Verification items for this drawing (mm, ordinates from the low corner). A direction names the side the tool comes from. Round coordinates to 2 decimals unless told otherwise and drop trailing zeros. Write each loop counter-clockwise with the first axis right and the second up, starting at its lowest first coordinate (ties: lowest second). Pieces come first, ordered by that corner, then holes.
Item 1: Scan lines: probe 1 along X at (y, z) = (4.5, 21); probe 2 along Y at (x, z) = (37.5, 40); probe 3 along X at (y, z) = (9, 9) (1 decimal). Record each from-to range of solid material in increasing order.
Item 2: Cross-section at D-D (x = 5). Enter the section's corners in (y, z), then the cut area to 3 significant figures.
Item 3: Cross-section at A-A (y = 5.5). Enter the section's corners in (x, z), then the cut area to 3 significant figures.
Item 4: Access from +Z, -Z, +X, -X, +Y, -Y to the whole of each face (thin tool, end or side, straight path). Record for the marked faces 1, 2 and 3.
Item 5: Draft check along X on the marked faces 4, 5 and 6. Enter one of: pulls with the +X half, pulls with the -X half, needs draft (parallel to the pull), parting line crosses it, or undercut.
Item 6: Cross-section at B-B (x = 26.25). Enter the section's corners in (y, z).
Item 7: Cross-section at C-C (z = 14). Enter the section's corners in (x, y) (1 decimal).
Item 8: Depth check by flat-ended pin: P1, Ø2.5, axis at x = 47, y = 14, coming from the -Z side; P2, Ø1, axis at x = 5, y = 14, coming from the +Z side; P3, Ø3.5, axis at y = 4.5, z = 6.5, coming from the -X side. Enter the tip coordinate at first touch or a pass-through.
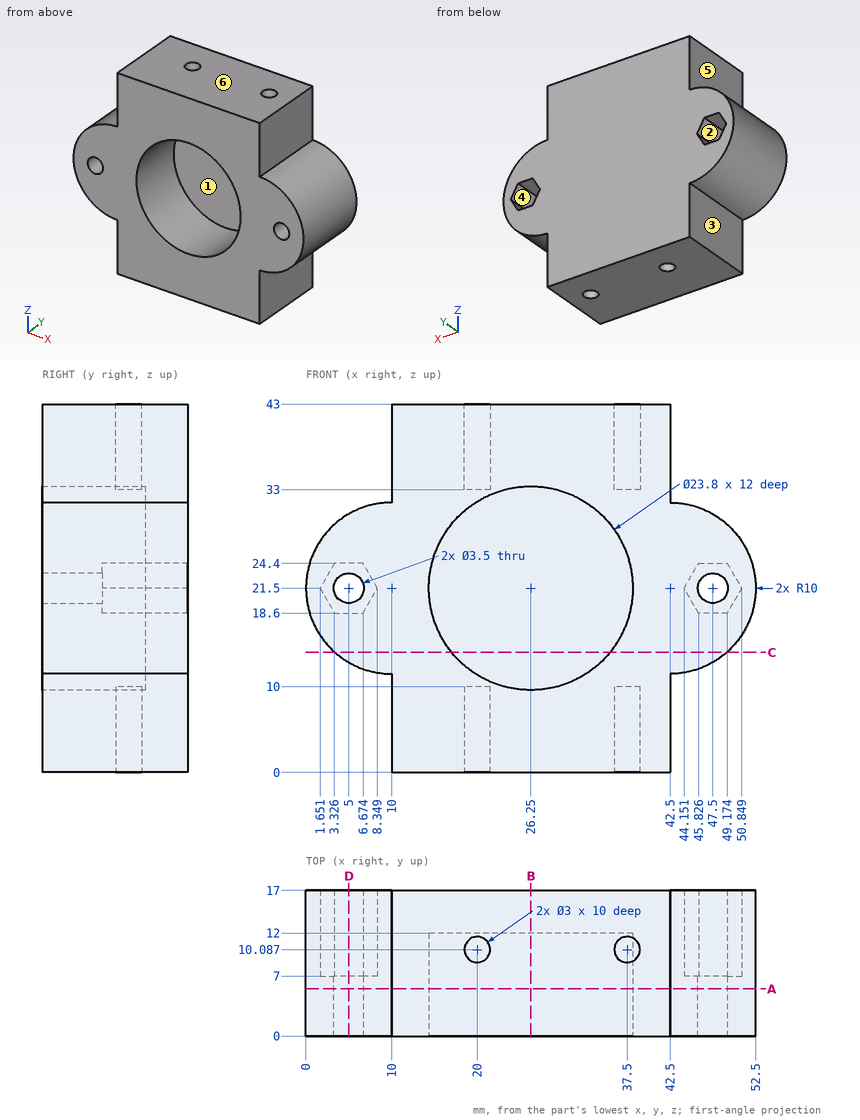
Resolved:
1. probe 1: x = 0.01 to 3.32, 6.68 to 14.36, 38.14 to 45.82, 49.18 to 52.49
1. probe 2: y = 0 to 8.59, 11.59 to 17
1. probe 3: x = 10 to 19, 21 to 36.5, 38.5 to 42.5
2. outline: (0, 12.84) - (17, 12.84) - (17, 18.6) - (7, 18.6) - (7, 19.75) - (0, 19.75) - close; (0, 23.25) - (7, 23.25) - (7, 24.4) - (17, 24.4) - (17, 30.16) - (0, 30.16) - close
2. area: 212 mm2
3. outline: (10, 0) - (42.5, 0) - (42.5, 11.5) arc R10 ccw to (42.5, 31.5) - (42.5, 43) - (10, 43) - (10, 31.5) arc R10 ccw to (10, 11.5) - close; hole circle Ø3.5 at (5, 21.5); hole circle Ø23.8 at (26.25, 21.5); hole circle Ø3.5 at (47.5, 21.5)
3. area: 1,250 mm2
4. face 1: -Y
4. face 2: +Y
4. face 3: -Z, -X, +Y, -Y
5. face 4: undercut
5. face 5: pulls with the -X half
5. face 6: needs draft
6. outline: (0, 0) - (17, 0) - (17, 43) - (0, 43) - (0, 33.4) - (12, 33.4) - (12, 9.6) - (0, 9.6) - close
7. outline: (3.4, 0) - (17, 0) - (17, 12) - (35.5, 12) - (35.5, 0) - (49.1, 0) - (49.1, 17) - (3.4, 17) - close
8. P1: stops at z = 12.04
8. P2: stops at z = 30.43
8. P3: stops at x = 10
